from build123d import *

# Parameters (mm, degrees)
BOSS_EXTRUDE1_DEPTH = 8.001
SKETCH2_W           = 20
SKETCH2_H           = 50.8
BOSS_EXTRUDE2_DEPTH = 12.7
FILLET1_R           = 7.62


with BuildPart() as part:
    # Sketch1 → Boss-Extrude1 (new body, symmetric)
    with BuildSketch(Plane.XY):
        Polygon((-28.575, 115.57), (-168.275, 115.57), (-168.275, 102.87), (-168.275, 0), (-168.275, -6.35), (0, -6.35), (0, 0), (-155.575, 0), (-155.575, 102.87), (-28.575, 102.87), align=None)
    extrude(amount=BOSS_EXTRUDE1_DEPTH, both=True)

    # Sketch2 → Boss-Extrude2 (add)
    with BuildSketch(Plane.XZ.offset(-102.87)):
        with Locations((-38.575, 0)):
            Rectangle(SKETCH2_W, SKETCH2_H)
    extrude(amount=-BOSS_EXTRUDE2_DEPTH)

    # Fillet1
    fillet1_edges = [part.edges().sort_by_distance(p)[0] for p in [
        (-155.575, 102.87, 0),
        (-155.575, 0, 0),
        (-168.275, -6.35, 0),
        (-168.275, 115.57, 0),
    ]]
    fillet(fillet1_edges, radius=FILLET1_R)


solid = part.part
Geometry check sheet. Reference: the model listing, model coordinates, mm. A direction names the side the tool comes from. Give positions to 0.01 mm unless a question says otherwise; leave off trailing zeros. Order: outer loops, then holes, each group sorted by start corner. A loop starts at its lowest first (then second) coordinate and runs counter-clockwise, first axis right, second up. Notation, with made-up numbers: (84.25, 74.25) - (117.25, 74.25) arc R21 cw to (117.25, 101.25) - close; hole circle Ø6 at (45, 13). An arc over 180 degrees is marked (long way). Use one line per item in the form item = value.
1) Access from +Z, -Z, +X, -X, +Y, -Y to the whole of each face (thin tool, end or side, straight path). Record for faces 4 (the face through (-48.575, 109, -17)), 5 (the face through (-168.275, 55, 0)), 6 (the face through (-28.575, 109, 0)), 7 (the face through (-153.28, 2.17, 0.11)), 8 (the face through (-48.575, 109, 17)).
Working result:
face_4 = -Z, -X, +Y, -Y
face_5 = +Z, -Z, -X, +Y, -Y
face_6 = +Z, -Z, +X, +Y
face_7 = +Z, -Z, +X
face_8 = +Z, -X, +Y, -Y
2) Draft check along Y on faces 1 (the face through (-73, 0, 0)), 2 (the face through (-81, 115.57, 0)), 3 (the face through (-159, 64, 8.001)). Enter one of: released by +Y, released by -Y, zero draft, split by the parting line, or undercut.
Working result:
face_1 = undercut
face_2 = released by +Y
face_3 = zero draft
3) Sectioned sample at A-A (x = -30.5). Record the boundary of the cut face in (y, z).
Working result:
outline = (-6.35, -8) - (0, -8) - (0, 8) - (-6.35, 8) - close; (102.87, -25.4) - (115.57, -25.4) - (115.57, 25.4) - (102.87, 25.4) - close
4) Depth check by flat-ended pin: pin 1 Ø3 at (y, z) = (44.5, -8) entering from +X (3 decimals); pin 2 Ø6 at (y, z) = (99.5, 12) entering from +X; pin 3 Ø14 at (y, z) = (108, 7) entering from +X (3 decimals); pin 4 Ø14 at (y, z) = (112, -12.5) entering from -X (3 decimals). Enter the tip coordinate at first touch or a pass-through.
Working result:
pin_1 = -155.575
pin_2 = through
pin_3 = -28.575
pin_4 = -168.275
5) Material ranges on probe 1 along Y at (x, z) = (-90, -0.5); probe 2 along Y at (x, z) = (-42, 17); probe 3 along Y at (x, z) = (-24, 2), recorded low to high. Write a range as from..to.
Working result:
probe_1 = -6.35..0, 102.87..115.57
probe_2 = 102.87..115.57
probe_3 = -6.35..0
6) Sectioned sample at D-D (y = 47). Record the boundary of the cut face in (x, z) (3 decimals).
Working result:
outline = (-168.275, -8.001) - (-155.575, -8.001) - (-155.575, 8.001) - (-168.275, 8.001) - close
7) Sectioned sample at C-C (x = -71.5). Record the boundary of the cut face in (y, z), and give its area (3 significant figures).
Working result:
outline = (-6.35, -8) - (0, -8) - (0, 8) - (-6.35, 8) - close; (102.87, -8) - (115.57, -8) - (115.57, 8) - (102.87, 8) - close
area = 305 mm^2
8) Sectioned sample at B-B (z = -1). Record the boundary of the cut face in (x, y) (3 decimals), and give its area (3 significant figures).
Working result:
outline = (-168.275, 1.27) arc R7.62 ccw to (-160.655, -6.35) - (0, -6.35) - (0, 0) - (-147.955, 0) arc R7.62 cw to (-155.575, 7.62) - (-155.575, 95.25) arc R7.62 cw to (-147.955, 102.87) - (-28.575, 102.87) - (-28.575, 115.57) - (-160.655, 115.57) arc R7.62 ccw to (-168.275, 107.95) - close
area = 4,150 mm^2
